Source: three-view drawing plus pictorial views. Frame: mm from the lowest corner of the part. Give positions to 0.01 mm unless a question says otherwise; leave off trailing zeros. Write each loop counter-clockwise with the first axis right and the second up, starting at its lowest first coordinate (ties: lowest second). Pieces come first, ordered by that corner, then holes.
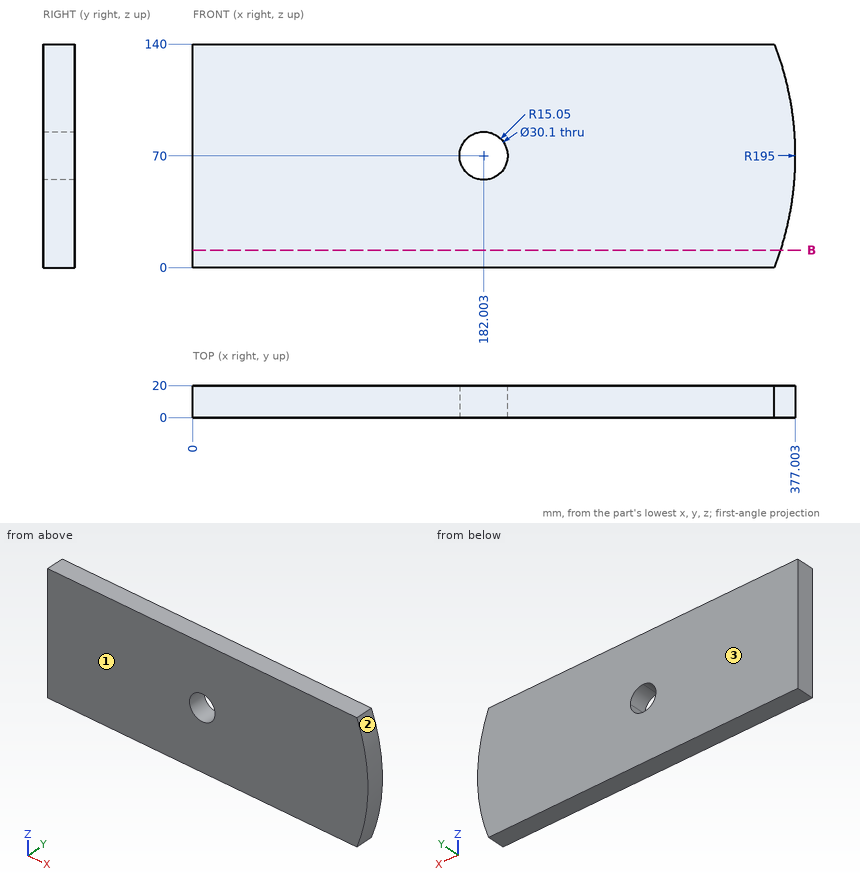
Q1. Pull-direction query (Y, two-part tool) for the marked faces 1, 2 and 3; classes: released by +Y, released by -Y, zero draft, split by the parting line, or undercut.
Filled sheet:
face 1: released by -Y
face 2: zero draft
face 3: released by +Y
Q2. Ray query, line 1 along X through (y, z) = (14.25, 79.5) (1 decimal); line 2 along X through (y, z) = (18, 102.5) (1 decimal); line 3 along X through (y, z) = (13.5, 96). Return the intervals inside material, ascending.
Filled sheet:
line 1: x = 0 to 170.3, 193.7 to 376.8
line 2: x = 0 to 374.3
line 3: x = 0 to 375.26
Q3. Pin query (flat end, axial travel): P1, Ø12, axis at y = 4, z = 20.5, coming from the +X side; P2, Ø3, axis at x = 269.5, z = 47.5, coming from the -Y side. Return the tip coordinate at first contact, or that it passes through.
Filled sheet:
P1: stops at x = 372.09
P2: stops at y = 0
Q4. Section B-B on z = 11. Output: boundary loops of the cut face in (x, y).
Filled sheet:
outline: (0, 0) - (367.86, 0) - (367.86, 20) - (0, 20) - close
